Check sheet for the modelled part. Datum: model origin and axes. Units: mm. Give positions to 0.01 mm unless a question says otherwise; leave off trailing zeros. Loops run counter-clockwise (first coordinate to the right, second up) from the corner with the lowest first, then second, coordinate; pieces in that order, holes last. Notation, with made-up numbers: M 74.5,-30.5 L 93.5,-30.5 A23 ccw 93.5,-19.5 Z; hole C -6.5,88.5 d8. An arc over 180 degrees is marked long. Write each question's results on one line, items separated by ' | '. Start each with the question number.
1. Go/stop test with flat-tipped pins: pin 1 (8 mm diameter, centred on y = 51, z = 13, fed in from +X); pin 2 (1.5 mm diameter, centred on x = 107.5, y = 47, fed in from -Z); pin 3 (10 mm diameter, centred on x = 257.5, y = 35.5, fed in from -Z). Record where each tip stops, or that it passes through.
2. Sectioned sample at B-B on y = 52. Record the cut outline in (x, z), and give its area (3 significant figures).
3. Draft check along Z on faces 1 (the flat face through (394, 32, 96)), 2 (the cylindrical face through (21.627, 31.552, 68.675)), 3 (the flat face through (377, 0, 20)). Enter one of: pulls with the +Z half, pulls with the -Z half, needs draft (parallel to the pull), parting line crosses it, or undercut.
4. Sectioned sample at C-C on z = -44. Record the cut outline in (x, y).
5. Sectioned sample at D-D on x = 626. Record the cut outline in (y, z).
6. Sectioned sample at A-A on z = 2.5. Record the cut outline in (x, y), and give its area (3 significant figures).
7. Material ranges on line 1 along X through (y, z) = (30, 34.5); line 2 along X through (y, z) = (19, 37.5); line 3 along Z through (x, y) = (549.5, 60.5), recorded low to high.
```python
from build123d import *

# Parameters (mm, degrees)
SKETCH1_R           = 72
BOSS_EXTRUDE2_DEPTH = 64


with BuildPart() as part:
    # Sketch1 → Boss-Extrude2 (new body)
    # profile 1 of 6: a face of its own
    with BuildSketch(Plane(origin=(0, 0, 0), x_dir=(1, 0, 0), z_dir=(0, 1, 0))):
        with BuildLine():
            ThreePointArc((0, 96), (-96, 0), (0, -96))
            ThreePointArc((0, -96), (67.882250994, -67.882250994), (96, 0))
            ThreePointArc((96, 0), (73.079350127, 62.252779738), (15.262321145, 94.779014308))
            Line((15.262321145, 94.779014308), (0, 96))
        make_face()
        with Locations(Location((0, 0, 0), (0, 0, 270))):
            Circle(SKETCH1_R, mode=Mode.SUBTRACT)
    # profile 2 of 6: a face of its own
    with BuildSketch(Plane(origin=(0, 0, 0), x_dir=(1, 0, 0), z_dir=(0, 1, 0))):
        with BuildLine():
            ThreePointArc((96, 0), (67.882250994, -67.882250994), (0, -96))
            Line((0, -96), (800, -96))
            ThreePointArc((800, -96), (736, -32), (800, 32))
            Line((800, 32), (15.262321145, 94.779014308))
            ThreePointArc((15.262321145, 94.779014308), (73.079350127, 62.252779738), (96, 0))
        make_face()
    # profile 3 of 6: a face of its own
    with BuildSketch(Plane(origin=(0, 0, 0), x_dir=(1, 0, 0), z_dir=(0, 1, 0))):
        with BuildLine():
            ThreePointArc((800, 32), (736, -32), (800, -96))
            Line((800, -96), (800, -80))
            ThreePointArc((800, -80), (752, -32), (800, 16))
            Line((800, 16), (800, 32))
        make_face()
    # profile 4 of 6: a face of its own
    with BuildSketch(Plane(origin=(0, 0, 0), x_dir=(1, 0, 0), z_dir=(0, 1, 0))):
        with BuildLine():
            Line((800, -80), (800, -96))
            ThreePointArc((800, -96), (845.254833996, -77.254833996), (864, -32))
            ThreePointArc((864, -32), (845.254833996, 13.254833996), (800, 32))
            Line((800, 32), (800, 16))
            ThreePointArc((800, 16), (833.941125497, 1.941125497), (848, -32))
            ThreePointArc((848, -32), (833.941125497, -65.941125497), (800, -80))
        make_face()
    # profile 5 of 6: a face of its own
    with BuildSketch(Plane(origin=(0, 0, 0), x_dir=(1, 0, 0), z_dir=(0, 1, 0))):
        with BuildLine():
            ThreePointArc((800, 32), (736, -32), (800, -96))
            Line((800, -96), (800, -80))
            ThreePointArc((800, -80), (752, -32), (800, 16))
            Line((800, 16), (800, 32))
        make_face()
    # profile 6 of 6: a face of its own
    with BuildSketch(Plane(origin=(0, 0, 0), x_dir=(1, 0, 0), z_dir=(0, 1, 0))):
        with BuildLine():
            Line((800, -80), (800, -96))
            ThreePointArc((800, -96), (845.254833996, -77.254833996), (864, -32))
            ThreePointArc((864, -32), (845.254833996, 13.254833996), (800, 32))
            Line((800, 32), (800, 16))
            ThreePointArc((800, 16), (833.941125497, 1.941125497), (848, -32))
            ThreePointArc((848, -32), (833.941125497, -65.941125497), (800, -80))
        make_face()
    extrude(amount=BOSS_EXTRUDE2_DEPTH)


solid = part.part
```
Output values:
1) pin 1: x = 862.22 | pin 2: z = -87.46 | pin 3: z = -75.8
2) outline: M 0,-96 L 800,-32 A64 ccw 800,96 L 0,96 A96 ccw Z; hole C 0,0 d144; hole C 800,32 d96 | area: 125,000 mm2
3) face 1: pulls with the +Z half | face 2: undercut | face 3: needs draft
4) outline: M -85.32,0 L -56.99,0 L -56.99,64 L -85.32,64 Z; M 56.99,0 L 650,0 L 650,64 L 56.99,64 Z
5) outline: M 0,-45.92 L 64,-45.92 L 64,96 L 0,96 Z
6) outline: M -95.97,0 L -71.96,0 L -71.96,64 L -95.97,64 Z; M 71.96,0 L 762.14,0 L 762.14,64 L 71.96,64 Z; M 837.86,0 L 856.8,0 L 856.8,64 L 837.86,64 Z | area: 46,900 mm2
7) line 1: -89.59 to -63.2, 63.2 to 752.07, 847.93 to 863.95 | line 2: -88.37 to -61.46, 61.46 to 752.32, 847.68 to 863.76 | line 3: -52.04 to 96
